Verification items for the finished model (mm, model axes). A direction names the side the tool comes from. Round coordinates to 2 decimals unless told otherwise and drop trailing zeros. Loops run counter-clockwise (first coordinate to the right, second up) from the corner with the lowest first, then second, coordinate; pieces in that order, holes last. Notation, with made-up numbers: (49.5, 61.5) -> (103.5, 61.5) arc R19 cw to (103.5, 88.5) -> close; hole circle Ø5 at (13.25, -25.5). An arc over 180 degrees is marked (long way). Write item = value, one per line.
Autodesk Inventor part; units mm, degrees
ref_plane "YZ Plane" through (0, 0, 0) normal (1, 0, 0) x (0, 1, 0)
ref_plane "XZ Plane" through (0, 0, 0) normal (0, 1, 0) x (-1, 0, 0)
ref_plane "XY Plane" through (0, 0, 0) normal (0, 0, 1) x (1, 0, 0)
sketch "Sketch1" plane through (0, 0, 0) normal (0, 0, 1) x (1, 0, 0)
  line L0 (-63.5, -66.5) -> (63.5, -66.5)
  line L1 (63.5, -66.5) -> (63.5, 66.5)
  line L2 (63.5, 66.5) -> (-63.5, 66.5)
  line L3 (-63.5, 66.5) -> (-63.5, -66.5)
  line L4 (-63.5, -66.5) -> (63.5, 66.5) construction
  line L5 (63.5, -66.5) -> (-63.5, 66.5) construction
  line L6 (-45.1, 66.5) -> (-24.9, 66.5)
  line L7 (-24.9, 66.5) -> (-24.9, 63.5)
  line L8 (-24.9, 63.5) -> (-45.1, 63.5)
  line L9 (-45.1, 63.5) -> (-45.1, 66.5)
  line L10 (-45.1, 66.5) -> (-24.9, 63.5) construction
  line L11 (-24.9, 66.5) -> (-45.1, 63.5) construction
  line L12 (-10.1, 66.5) -> (10.1, 66.5)
  line L13 (10.1, 66.5) -> (10.1, 63.5)
  line L14 (10.1, 63.5) -> (-10.1, 63.5)
  line L15 (-10.1, 63.5) -> (-10.1, 66.5)
  line L16 (-10.1, 66.5) -> (10.1, 63.5) construction
  line L17 (10.1, 66.5) -> (-10.1, 63.5) construction
  line L18 (24.9, 66.5) -> (45.1, 66.5)
  line L19 (45.1, 66.5) -> (45.1, 63.5)
  line L20 (45.1, 63.5) -> (24.9, 63.5)
  line L21 (24.9, 63.5) -> (24.9, 66.5)
  line L22 (24.9, 66.5) -> (45.1, 63.5) construction
  line L23 (45.1, 66.5) -> (24.9, 63.5) construction
  line L24 (-63.5, 39) -> (-60.5, 39)
  line L25 (-60.5, 39) -> (-60.5, 24) construction
  line L26 (-60.5, 24) -> (-63.5, 24)
  line L27 (-63.5, 24) -> (-63.5, 39)
  line L28 (-63.5, 39) -> (-60.5, 24) construction
  line L29 (-60.5, 39) -> (-63.5, 24) construction
  line L30 (-63.5, 9) -> (-60.5, 9)
  line L31 (-60.5, 9) -> (-60.5, -6) construction
  line L32 (-60.5, -6) -> (-63.5, -6)
  line L33 (-63.5, -6) -> (-63.5, 9)
  line L34 (-63.5, 9) -> (-60.5, -6) construction
  line L35 (-60.5, 9) -> (-63.5, -6) construction
  line L36 (-63.5, -21) -> (-60.5, -21)
  line L37 (-60.5, -21) -> (-60.5, -36) construction
  line L38 (-60.5, -36) -> (-63.5, -36)
  line L39 (-63.5, -36) -> (-63.5, -21)
  line L40 (-63.5, -21) -> (-60.5, -36) construction
  line L41 (-60.5, -21) -> (-63.5, -36) construction
  line L42 (-60.5, 39) -> (-60.5, 66.5)
  line L43 (-60.5, 24) -> (-60.5, 9)
  line L44 (-60.5, -6) -> (-60.5, -21)
  line L45 (-60.5, 51) -> (-40.5, 51)
  line L46 (-40.5, 51) -> (-40.5, 56)
  line L47 (-40.5, 56) -> (-60.5, 56)
  line L48 (-60.5, 56) -> (-60.5, 51)
  line L49 (-60.5, 51) -> (-40.5, 56) construction
  line L50 (-40.5, 51) -> (-60.5, 56) construction
  line L51 (-60.5, -64) -> (-40.5, -64)
  line L52 (-40.5, -66.5) -> (-40.5, -59)
  line L53 (-40.5, -59) -> (-60.5, -59)
  line L54 (-60.5, -59) -> (-60.5, -64)
  line L55 (-60.5, -64) -> (-40.5, -59) construction
  line L56 (-40.5, -64) -> (-60.5, -59) construction
  line L57 (-60.5, 48.5) -> (-55.5, 48.5)
  line L58 (-55.5, 48.5) -> (-55.5, 58.5)
  line L59 (-55.5, 58.5) -> (-60.5, 58.5)
  line L60 (-60.5, 58.5) -> (-60.5, 48.5)
  line L61 (-60.5, 48.5) -> (-55.5, 58.5) construction
  line L62 (-55.5, 48.5) -> (-60.5, 58.5) construction
  line L63 (-60.5, -66.5) -> (-55.5, -66.5)
  line L64 (-55.5, -66.5) -> (-55.5, -56.5)
  line L65 (-55.5, -56.5) -> (-60.5, -56.5)
  line L66 (-60.5, -56.5) -> (-60.5, -66.5)
  line L67 (-60.5, -66.5) -> (-55.5, -56.5) construction
  line L68 (-55.5, -66.5) -> (-60.5, -56.5) construction
  line L69 (-60.5, -36) -> (-60.5, -66.5)
  point P0 (0, 0)
  point P1 (-35, 65)
  point P2 (0, 65)
  point P3 (35, 65)
  point P4 (0, 66.5)
  point P5 (-62, 31.5)
  point P6 (-62, 1.5)
  point P7 (-62, -28.5)
  point P8 (45.1, 66.5)
  point P9 (24.9, 66.5)
  point P10 (10.1, 66.5)
  point P11 (-63.5, -36)
  point P12 (-63.5, -6)
  point P13 (-63.5, 9)
  point P14 (-63.5, 39)
  point P15 (-50.5, 53.5)
  point P16 (-50.5, -61.5)
  point P17 (-60.5, 56)
  point P18 (-60.5, 51)
  point P19 (-58, 53.5)
  point P20 (-40.5, 53.5)
  point P21 (-58, -61.5)
  point P22 (-55.5, 56)
  point P23 (-55.5, 51)
  point P24 (-55.5, -59)
  point P25 (-55.5, -64)
  dimension "d0" = 127
  dimension "d1" = 133
  dimension "d2" = 3
  dimension "d3" = 20.2
  dimension "d5" = 3
  dimension "d6" = 20.2
  dimension "d9" = 3
  dimension "d10" = 20.2
  dimension "d13" = 35
  dimension "d14" = 35
  dimension "d15" = 15
  dimension "d16" = 3
  dimension "d17" = 15
  dimension "d18" = 3
  dimension "d19" = 15
  dimension "d20" = 3
  dimension "d21" = 30
  dimension "d22" = 30
  dimension "d23" = 35
  dimension "d31" = 5
  dimension "d32" = 20
  dimension "d33" = 5
  dimension "d34" = 20
  dimension "d35" = 5
  dimension "d36" = 13
  dimension "d37" = 5
  dimension "d38" = 10
  dimension "d39" = 5
  dimension "d40" = 10
extrude "Extrusion1" add sketch "Sketch1" along normal blind 3 contours L3 L38 L69 L66 L54 L0 | L66 L51 L64 L0 | L3 L36 L44 L32 L30 L43 L26 L24 L42 L57 L58 L45 L46 L47 L59 L2 L9 L8 L7 L15 L14 L13 L21 L20 L19 L1 L0 L52 L53 L64 L65 L69 L38 | L64 L51 L52 L0 | L54 L53 L64 L51 | L3 L32 L44 L36 | L64 L53 L52 L51 | L66 L65 L64 L53 | L3 L26 L43 L30 | L3 L2 L42 L24 | L42 L45 L58 L57 | L59 L58 L47 L42 | L42 L47 L58 L45 | L58 L47 L46 L45
extrude "Extrusion2" cut sketch "Sketch1" along normal through all contours L3 L38 L69 L66 L54 L0 | L66 L51 L64 L0 | L64 L51 L52 L0 | L54 L53 L64 L51 | L3 L32 L44 L36 | L64 L53 L52 L51 | L66 L65 L64 L53 | L3 L26 L43 L30 | L3 L2 L42 L24 | L42 L45 L58 L57 | L59 L58 L47 L42 | L42 L47 L58 L45 | L58 L47 L46 L45
mirror "Mirror1" about plane through (0, 0, 0) normal (1, 0, 0) of "Extrusion2"
equation "\"d5\" = d2"
equation "\"d6\" = d3"
equation "\"d9\" = d2"
equation "\"d10\" = d11"
equation "\"d16\" = d2"
equation "\"d17\" = d15"
equation "\"d18\" = d16"
equation "\"d19\" = d17"
equation "\"d20\" = d18"
equation "\"d33\" = d31"
equation "\"d34\" = d32"
properties part number "bed_acrylic_floor"
(1) Set-up check for faces 5 (the face through (24.9, 65, 1)), 6 (the face through (62, 9, 1)), 7 (the face through (-62, 24, 1)), 8 (the face through (-60.5, -46, 1)): record each of +Z, -Z, +X, -X, +Y, -Y from which the full face is reachable in a straight line by a thin tool's end or side.
Filled sheet:
face_5 = +Z, -Z, +Y
face_6 = +Z, -Z, +X
face_7 = +Z, -Z, -X
face_8 = +Z, -Z, -X, -Y
(2) Draft check along Y on faces 1 (the face through (45.1, 65, 1)), 2 (the face through (-58, -56.5, 1)), 3 (the face through (-60.5, 17, 1)), 4 (the face through (-58, 58.5, 1)). Enter one of: released by +Y, released by -Y, zero draft, split by the parting line, or undercut.
Filled sheet:
face_1 = zero draft
face_2 = released by -Y
face_3 = undercut
face_4 = undercut
(3) Material ranges on probe 1 along Y at (x, z) = (42, 2.3); probe 2 along Y at (x, z) = (54.5, 0.95); probe 3 along X at (y, z) = (55, 2.35), recorded low to high. Write a range as from..to.
Filled sheet:
probe_1 = -59..51, 56..63.5
probe_2 = -59..51, 56..66.5
probe_3 = -40.5..40.5
(4) Sectioned sample at A-A, the plane x = 34. Record the cut outline in (y, z), and give its area (3 significant figures).
Filled sheet:
outline = (-66.5, 0) -> (63.5, 0) -> (63.5, 3) -> (-66.5, 3) -> close
area = 390 mm2
(5) Go/stop test with flat-tipped pins: pin 1 Ø12 at (x, y) = (18, -23.5) entering from -Z; pin 2 Ø0.9 at (y, z) = (53, 1.5) entering from -X; pin 3 Ø0.9 at (y, z) = (17.5, 1.5) entering from +X; pin 4 Ø1.5 at (y, z) = (64.5, 1.5) entering from -X. Record where each tip stops, or that it passes through.
Filled sheet:
pin_1 = 0
pin_2 = -40.5
pin_3 = 60.5
pin_4 = -60.5
(6) Sectioned sample at B-B, the plane y = 16. Record the cut outline in (x, z), and give its area (3 significant figures).
Filled sheet:
outline = (-60.5, 0) -> (60.5, 0) -> (60.5, 3) -> (-60.5, 3) -> close
area = 363 mm2
